from build123d import *

# Parameters (mm, degrees)
SKETCH1_W                    = 44.01968481
SKETCH1_H                    = 69.878571894
BOSS_EXTRUDE1_DEPTH          = 3.175
SKETCH3_W                    = 18.555037993
SKETCH3_H                    = 36.867111451
CUT_EXTRUDE1_DEPTH           = 3.175
EDGE_FLANGE1_STRIP_W         = 19.05
EDGE_FLANGE1_STRIP_H         = 3.175
EDGE_FLANGE1_STRIP_CUT_DEPTH = 25.464646817
EDGE_FLANGE1_DEPTH           = 25.464646817
SKETCH22_W                   = 44.01968481
SKETCH22_H                   = 20.04943399
CUT_EXTRUDE2_DEPTH           = 3.175
FILLET1_R                    = 3
SKETCH23_R                   = 3.008539127
SKETCH23_R_2                 = 3
CUT_EXTRUDE3_DEPTH           = 3.175
SKETCH24_R                   = 1.724090174
SKETCH24_R_2                 = 1.754985839
CUT_EXTRUDE4_DEPTH           = 3.175


# Sheet-metal steps are written as plain solids
with BuildPart() as part:
    # Sketch1 → Boss-Extrude1 (new body)
    with BuildSketch(Plane.XY):
        Rectangle(SKETCH1_W, SKETCH1_H)
    extrude(amount=BOSS_EXTRUDE1_DEPTH)

    # Sketch3 → Cut-Extrude1 (cut)
    with BuildSketch(Plane.XY.offset(3.175)):
        with Locations((12.732323409, 16.505730222)):
            Rectangle(SKETCH3_W, SKETCH3_H)
    extrude(amount=-CUT_EXTRUDE1_DEPTH, mode=Mode.SUBTRACT)

    # Edge-Flange1 strip (across the edge) → Edge-Flange1 strip cut (cut)
    with BuildSketch(Plane(origin=(-22.009842405, 34.939285947, 0), x_dir=(0, -1, 0), z_dir=(1, 0, 0))):
        with Locations((-3.175, -1.5875)):
            Rectangle(EDGE_FLANGE1_STRIP_W, EDGE_FLANGE1_STRIP_H)
    extrude(amount=EDGE_FLANGE1_STRIP_CUT_DEPTH, mode=Mode.SUBTRACT)

    # Edge-Flange1 section (across the edge) → Edge-Flange1 (add)
    with BuildSketch(Plane(origin=(-22.009842405, 34.939285947, 0), x_dir=(0, -1, 0), z_dir=(1, 0, 0))):
        with BuildLine():
            Line((0, 3.175), (0, 20.35))
            Line((0, 20.35), (3.175, 20.35))
            Line((3.175, 20.35), (3.175, 3.175))
            ThreePointArc((3.175, 3.175), (4.10493597, 0.92993597), (6.35, 0))
            Line((6.35, 0), (6.35, -3.175))
            ThreePointArc((6.35, -3.175), (1.859871939, -1.315128061), (0, 3.175))
        make_face()
    extrude(amount=EDGE_FLANGE1_DEPTH)

    # Sketch22 → Cut-Extrude2 (cut)
    with BuildSketch(Plane.XY.offset(3.175)):
        with Locations((0, -24.914568952)):
            Rectangle(SKETCH22_W, SKETCH22_H)
    extrude(amount=-CUT_EXTRUDE2_DEPTH, mode=Mode.SUBTRACT)

    # Fillet1
    fillet1_edges = [part.edges().sort_by_distance(p)[0] for p in [
        (22.009842405, -1.927825504, 1.5875),
        (3.454804412, -1.927825504, 1.5875),
        (-22.009842405, 33.351785947, -20.35),
        (3.454804412, 33.351785947, -20.35),
        (-22.009842405, -14.889851957, 1.5875),
        (22.009842405, -14.889851957, 1.5875),
    ]]
    fillet(fillet1_edges, radius=FILLET1_R)

    # Sketch23 → Cut-Extrude3 (cut)
    with BuildSketch(Plane.XY.offset(3.175)):
        with Locations((-16.805425884, -9.867122138)):
            Circle(SKETCH23_R)
        with Locations((16.248443226, -9.867122138)):
            Circle(SKETCH23_R_2)
    extrude(amount=-CUT_EXTRUDE3_DEPTH, mode=Mode.SUBTRACT)

    # Sketch24 → Cut-Extrude4 (cut)
    with BuildSketch(Plane(origin=(0, 34.939285947, 0), x_dir=(1, 0, 0), z_dir=(0, 1, 0))):
        with Locations(Location((-9.277518997, 9.296029356, 0), (0, 0, 270))):
            Circle(SKETCH24_R)
        with Locations(Location((-9.277518997, 14.371964171, 0), (0, 0, 270))):
            Circle(SKETCH24_R_2)
    extrude(amount=-CUT_EXTRUDE4_DEPTH, mode=Mode.SUBTRACT)


solid = part.part
Part model, mm, in its own coordinate system. A direction names the side the tool comes from. Coordinates: 2 decimals unless noted, no trailing zeros. Order: outer loops, then holes, each group sorted by start corner. A loop starts at its lowest first (then second) coordinate and runs counter-clockwise, first axis right, second up. Notation, with made-up numbers: M 17.25,0 L 28.25,0 A19 ccw 28.25,15 Z; hole C -14,-31 d11. An arc over 180 degrees is marked long. Use a Markdown table: item, result.
(1) Pull direction X, two halves, no side cores. Call faces 3 (the flat face through (3.455, 21.7, 0.5)), 4 (the flat face through (-5, 2, 0)), 5 (the cylindrical face through (-19.19, -11.7, 1.61)): released by +X, released by -X, zero draft, split by the parting line, or undercut.
A:
| item | result |
|---|---|
| face 3 | released by +X |
| face 4 | zero draft |
| face 5 | undercut |
(2) Tool access for faces 1 (the cylindrical face through (-9.456, 33.03, 1.364)), 2 (the flat face through (-9, 31.764, -12)): list every direction of +Z, -Z, +X, -X, +Y, -Y with a clear straight run to the whole face (end or side of a thin tool).
A:
| item | result |
|---|---|
| face 1 | +Z, +X, -X, +Y |
| face 2 | -Z, +X, -X, -Y |
(3) Cut at B-B on z = -14. Write the cut outline in (x, y), then the cut area to 3 significant figures.
A:
| item | result |
|---|---|
| outline | M -22.01,31.76 L -10.99,31.76 L -10.99,34.94 L -22.01,34.94 Z; M -7.56,31.76 L 3.45,31.76 L 3.45,34.94 L -7.56,34.94 Z |
| area | 70.0 mm^2 |
(4) Cut at D-D on z = -10.25. Write the cut outline in (x, y), then the cut area to 3 significant figures.
A:
| item | result |
|---|---|
| outline | M -22.01,31.76 L -10.71,31.76 L -10.71,34.94 L -22.01,34.94 Z; M -7.84,31.76 L 3.45,31.76 L 3.45,34.94 L -7.84,34.94 Z |
| area | 71.7 mm^2 |
(5) Cut at C-C on y = 24.5. Write the cut outline in (x, z) (3 decimals).
A:
| item | result |
|---|---|
| outline | M -22.01,0 L 3.455,0 L 3.455,3.175 L -22.01,3.175 Z |
(6) Flat gauge pins, fed straight in: pin 1 (8 mm diameter, centred on y = 5.5, z = -4.5, fed in from +X); pin 2 (3.5 mm diameter, centred on x = 9.5, z = 1, fed in from +Y); pin 3 (8.5 mm diameter, centred on x = -10, z = -11, fed in from -Y); pin 4 (2 mm diameter, centred on x = -10, y = -5.5, fed in from -Z). Where does each tip first touch, or does it go through?
A:
| item | result |
|---|---|
| pin 1 | passes through |
| pin 2 | stops at y = -1.93 |
| pin 3 | stops at y = 31.76 |
| pin 4 | stops at z = 0 |
(7) Probe L1, parallel to Y at x = -19, z = -12.75; L2, parallel to Z at x = -7, y = 22.5 (3 decimals); L3, parallel to Y at x = -19.5, z = 1. List the from-to ranges inside material, lowest first.
A:
| item | result |
|---|---|
| L1 | y = 31.76 to 34.94 |
| L2 | z = 0 to 3.175 |
| L3 | y = -14.85 to -11.21, -8.53 to 33.37 |
(8) Cut at A-A on x = -3. Write the cut outline in (y, z) (3 decimals).
A:
| item | result |
|---|---|
| outline | M -14.89,0 L 28.589,0 A3.175 cw 31.764,-3.175 L 31.764,-20.35 L 34.939,-20.35 L 34.939,-3.175 A6.35 ccw 28.589,3.175 L -14.89,3.175 Z |
